For this review, take the finished solid that the model builds, in its own axes (mm). A direction names the side the tool comes from. Give positions to 0.01 mm unless a question says otherwise; leave off trailing zeros. Order: outer loops, then holes, each group sorted by start corner. A loop starts at its lowest first (then second) coordinate and runs counter-clockwise, first axis right, second up. Notation, with made-up numbers: (-17.5, 39.5) - (15.5, 39.5) arc R15 ccw to (15.5, 59.5) - close; hole circle Ø8 at (89, 20). An arc over 180 degrees is marked (long way). One line per item, written item: value.
```python
from build123d import *

# Parameters (mm, degrees)
BOSS_EXTRUDE1_DEPTH = 38.1
CUT_EXTRUDE1_DEPTH  = 98.457965419
SHELL1_START        = -38.1
SHELL1_DEPTH        = 75.35333418
FILLET1_R           = 17.78


# Read off the part's stored shape, not the designer's step: Shell1
with BuildPart() as part:
    # Sketch1 → Boss-Extrude1 (new, symmetric)
    with BuildSketch(Plane.XY):
        Polygon((-33.198119966, 25.4), (-33.198119966, -25.4), (33.198119966, -50.887128572), (33.198119966, -0.087128572), align=None)
    extrude(amount=BOSS_EXTRUDE1_DEPTH, both=True)

    # Sketch2 → Cut-Extrude1 (cut, through all)
    with BuildSketch(Plane.XY.offset(38.1)):
        Polygon((16.599059983, -44.515346429), (33.198119966, -33.107128572), (33.198119966, -50.887128572), align=None)
        Polygon((-16.599059983, 19.028217857), (-33.198119966, 25.4), (-33.198119966, 7.62), align=None)
    extrude(amount=-CUT_EXTRUDE1_DEPTH, mode=Mode.SUBTRACT)

    # Shell1 outline → Shell1 (cut)
    with BuildSketch(Plane.XY.offset(SHELL1_START)):
        Polygon((31.928119966, -0.506523102), (-16.486612201, 18.078151343), (-32.351454146, 7.174547563), (-32.351454146, -24.818102704), (16.486612201, -43.565279915), (31.928119966, -32.952625656), align=None)
    extrude(amount=SHELL1_DEPTH, mode=Mode.SUBTRACT)

    # Fillet1
    # the kernel refuses this fillet: 17.78 mm, written as the material it adds along each edge
    with BuildSketch(Plane(origin=(-14.571454146, -2.179962965, 19.47333418), x_dir=(-0.5664062369240325, 0.8241261886225658, 0), z_dir=(0, 0, 1))) as fillet1_piece_1_section:
        Polygon((0, 0), (FILLET1_R * 1.02, 0), (FILLET1_R * 1.02, FILLET1_R * 0.536647960523), (FILLET1_R * 0.577734361663, FILLET1_R * 0.840608712395), align=None)
    fillet1_piece_1 = extrude(amount=FILLET1_R * 1.02, mode=Mode.PRIVATE)
    fillet1_piece_1 = fillet1_piece_1 - Plane(origin=(-14.571454146, -2.179962965, 19.47333418), x_dir=(0.8849876374628157, -0.4656145203255411, 0), z_dir=(0, 0, 1)) * Sphere(FILLET1_R, mode=Mode.PRIVATE)
    add(fillet1_piece_1)
    with BuildSketch(Plane(origin=(-14.571454146, -12.59824726, 19.47333418), x_dir=(-1, 0, 0), z_dir=(0, 0, 1))) as fillet1_piece_2_section:
        Polygon((0, 0), (FILLET1_R * 1.02, 0), (FILLET1_R * 1.02, FILLET1_R * 0.701026577777), (FILLET1_R * 0.365535308531, FILLET1_R * 0.952252035029), align=None)
    fillet1_piece_2 = extrude(amount=FILLET1_R * 1.02, mode=Mode.PRIVATE)
    fillet1_piece_2 = fillet1_piece_2 - Plane(origin=(-14.571454146, -12.59824726, 19.47333418), x_dir=(0.8241261886205663, 0.5664062369269417, 0), z_dir=(0, 0, 1)) * Sphere(FILLET1_R, mode=Mode.PRIVATE)
    add(fillet1_piece_2)
    with BuildSketch(Plane(origin=(14.148119966, -12.726378546, 19.47333418), x_dir=(0.35836794954893786, 0.9335804264958054, 0), z_dir=(0, 0, 1))) as fillet1_piece_3_section:
        Polygon((0, 0), (FILLET1_R * 1.02, 0), (FILLET1_R * 1.02, -FILLET1_R * 0.701026577771), (FILLET1_R * 0.36553530854, -FILLET1_R * 0.952252035026), align=None)
    fillet1_piece_3 = extrude(amount=FILLET1_R * 1.02, mode=Mode.PRIVATE)
    fillet1_piece_3 = fillet1_piece_3 - Plane(origin=(14.148119966, -12.726378546, 19.47333418), x_dir=(-0.824126188623119, -0.5664062369232272, 0), z_dir=(0, 0, 1)) * Sphere(FILLET1_R, mode=Mode.PRIVATE)
    add(fillet1_piece_3)
    with BuildSketch(Plane(origin=(-14.125206416, -1.873265397, 19.47333418), x_dir=(0.35836794954893786, 0.9335804264958054, 0), z_dir=(0, 0, 1))) as fillet1_piece_4_section:
        Polygon((0, 0), (FILLET1_R * 1.02, 0), (FILLET1_R * 1.02, FILLET1_R * 0.536647960524), (FILLET1_R * 0.577734361661, FILLET1_R * 0.840608712396), align=None)
    fillet1_piece_4 = extrude(amount=FILLET1_R * 1.02, mode=Mode.PRIVATE)
    fillet1_piece_4 = fillet1_piece_4 - Plane(origin=(-14.125206416, -1.873265397, 19.47333418), x_dir=(0.11753739745542074, -0.9930684569552123, 0), z_dir=(0, 0, 1)) * Sphere(FILLET1_R, mode=Mode.PRIVATE)
    add(fillet1_piece_4)
    with BuildSketch(Plane(origin=(-32.351454146, -2.179962965, 37.25333418), x_dir=(0, 0, -1), z_dir=(0, -1, 0))) as fillet1_piece_5:
        with BuildLine():
            CenterArc((FILLET1_R, FILLET1_R), FILLET1_R, 180, 90)
            Line((0, FILLET1_R), (0, 0))
            Line((0, 0), (FILLET1_R, 0))
        make_face()
    extrude(amount=10.418284295)
    with BuildSketch(Plane(origin=(-20.943236289, -29.197307243, 37.25333418), x_dir=(0, 0, -1), z_dir=(0.9335804264990358, -0.3583679495405224, 0))) as fillet1_piece_6_section:
        with BuildLine():
            CenterArc((FILLET1_R, FILLET1_R), FILLET1_R, 180, 90)
            Line((0, FILLET1_R), (0, 0))
            Line((0, 0), (FILLET1_R, 0))
        make_face()
    fillet1_piece_6 = extrude(amount=84.542794822, mode=Mode.PRIVATE)
    fillet1_piece_6 = split(fillet1_piece_6, bisect_by=Plane(origin=(10.612775851, -47.602255792, 33.386694553), z_dir=(-0.5664062369254325, 0.8241261886216036, 0)), keep=Keep.TOP, mode=Mode.PRIVATE)
    fillet1_piece_6 = split(fillet1_piece_6, bisect_by=Plane(origin=(31.928119966, -33.018136408, 33.386694553), z_dir=(-1, 0, 0)), keep=Keep.TOP, mode=Mode.PRIVATE)
    add(fillet1_piece_6)
    with BuildSketch(Plane(origin=(31.928119966, -77.402625656, 37.25333418), x_dir=(0, 0, -1), z_dir=(0, 1, 0))) as fillet1_piece_7_section:
        with BuildLine():
            CenterArc((FILLET1_R, FILLET1_R), FILLET1_R, 180, 90)
            Line((0, FILLET1_R), (0, 0))
            Line((0, 0), (FILLET1_R, 0))
        make_face()
    fillet1_piece_7 = extrude(amount=64.67624711, mode=Mode.PRIVATE)
    fillet1_piece_7 = split(fillet1_piece_7, bisect_by=Plane(origin=(19.754469789, -44.819692915, 33.477432333), z_dir=(0.3583679495405224, 0.9335804264990358, 0)), keep=Keep.TOP, mode=Mode.PRIVATE)
    fillet1_piece_7 = split(fillet1_piece_7, bisect_by=Plane(origin=(33.035848264, -32.191305089, 33.477432333), z_dir=(-0.5664062369254325, 0.8241261886216036, 0)), keep=Keep.TOP, mode=Mode.PRIVATE)
    add(fillet1_piece_7)
    with BuildSketch(Plane(origin=(-32.351454146, -24.818102704, -38.1), x_dir=(0, 1, 0), z_dir=(0, 0, 1))) as fillet1_piece_8:
        with BuildLine():
            CenterArc((FILLET1_R * 0.687280958605, -FILLET1_R), FILLET1_R, 90, 69)
            Line((-FILLET1_R * 0.246299467894, -FILLET1_R * 0.641632050459), (0, 0))
            Line((0, 0), (FILLET1_R * 0.687280958605, 0))
        make_face()
    extrude(amount=57.57333418)
    with BuildSketch(Plane(origin=(-32.351454146, 7.174547563, -38.1), x_dir=(0.8241261886225659, 0.5664062369240322, 0), z_dir=(0, 0, 1))) as fillet1_piece_9:
        with BuildLine():
            CenterArc((FILLET1_R * 0.526125451493, -FILLET1_R), FILLET1_R, 90, 55.5)
            Line((-FILLET1_R * 0.29800073713, -FILLET1_R * 0.433593763076), (0, 0))
            Line((0, 0), (FILLET1_R * 0.526125451493, 0))
        make_face()
    extrude(amount=57.57333418)
    with BuildSketch(Plane(origin=(16.486612201, -43.565279915, -38.1), x_dir=(-0.933580426499036, 0.3583679495405219, 0), z_dir=(0, 0, 1))) as fillet1_piece_10:
        with BuildLine():
            CenterArc((FILLET1_R * 0.526125451489, -FILLET1_R), FILLET1_R, 90, 55.5)
            Line((-FILLET1_R * 0.29800073713, -FILLET1_R * 0.433593763072), (0, 0))
            Line((0, 0), (FILLET1_R * 0.526125451489, 0))
        make_face()
    extrude(amount=75.35333418)
    with BuildSketch(Plane(origin=(31.928119966, -32.952625656, -38.1), x_dir=(-0.8241261886216035, -0.5664062369254323, 0), z_dir=(0, 0, 1))) as fillet1_piece_11:
        with BuildLine():
            CenterArc((FILLET1_R * 0.526125451492, -FILLET1_R), FILLET1_R, 90, 55.5)
            Line((-FILLET1_R * 0.29800073713, -FILLET1_R * 0.433593763075), (0, 0))
            Line((0, 0), (FILLET1_R * 0.526125451492, 0))
        make_face()
    extrude(amount=75.35333418)
    with BuildSketch(Plane(origin=(-16.486612201, 18.078151343, -38.1), x_dir=(0.9335804264958054, -0.35836794954893825, 0), z_dir=(0, 0, 1))) as fillet1_piece_12:
        with BuildLine():
            CenterArc((FILLET1_R * 0.526125451494, -FILLET1_R), FILLET1_R, 90, 55.5)
            Line((-FILLET1_R * 0.29800073713, -FILLET1_R * 0.433593763078), (0, 0))
            Line((0, 0), (FILLET1_R * 0.526125451494, 0))
        make_face()
    extrude(amount=57.57333418)
    with BuildSketch(Plane(origin=(31.928119966, -0.506523102, -38.1), x_dir=(-0.9335804264958055, 0.3583679495489376, 0), z_dir=(0, 0, 1))) as fillet1_piece_13:
        with BuildLine():
            CenterArc((FILLET1_R * 0.687280958599, FILLET1_R), FILLET1_R, 201, 69)
            Line((-FILLET1_R * 0.246299467897, FILLET1_R * 0.641632050451), (0, 0))
            Line((0, 0), (FILLET1_R * 0.687280958599, 0))
        make_face()
    extrude(amount=57.57333418)
    with BuildSketch(Plane(origin=(20.519902109, 3.872681437, 37.25333418), x_dir=(0, 0, -1), z_dir=(-0.9335804264958054, 0.35836794954893786, 0))) as fillet1_piece_14:
        with BuildLine():
            CenterArc((FILLET1_R, FILLET1_R), FILLET1_R, 180, 90)
            Line((0, FILLET1_R), (0, 0))
            Line((0, 0), (FILLET1_R, 0))
        make_face()
    extrude(amount=30.284832008)
    with BuildSketch(Plane(origin=(-24.195909309, 12.779698237, 37.25333418), x_dir=(0, 0, -1), z_dir=(-0.8241261886225658, -0.5664062369240325, 0))) as fillet1_piece_15:
        with BuildLine():
            CenterArc((FILLET1_R, FILLET1_R), FILLET1_R, 180, 90)
            Line((0, FILLET1_R), (0, 0))
            Line((0, 0), (FILLET1_R, 0))
        make_face()
    extrude(amount=0.541479856)


solid = part.part
```
(1) For P1, Ø10, axis at x = -16.5, y = -3, coming from the -Z side; P2, Ø17.5, axis at x = -4, y = -10, coming from the -Z side; P3, Ø2, axis at x = -20.5, z = 18.5, coming from the -Y side; P4, Ø10, axis at x = 14, y = 5, coming from the -Z side, all flat-tipped, find the tip position at first contact; note any pin that passes through.
Answers below:
P1: stops at z = 35.85
P2: stops at z = 36.6
P3: stops at y = -30.66
P4: stops at z = -38.1
(2) Draft analysis for pull direction X (two halves, no side actions). For faces 1 (the face through (31.928, -18, -10)), 2 (the face through (24.782, -38.891, 0.533)), 3 (the face through (0, -12, 38.1)), state which applies: pulls with the +X half, pulls with the -X half, needs draft (parallel to the pull), parting line crosses it, or undercut.
Answers below:
face 1: undercut
face 2: pulls with the +X half
face 3: needs draft
(3) Wall thickness on line 1 (Y direction, x = 0, z = 33); line 2 (X direction, y = -11.5, z = 4.5); line 3 (Y direction, x = -2, z = -23.5): over which ranges is each line inside the solid? List them lowest first. Write a range as from..to.
Answers below:
line 1: y = -38.14..-30.55, 5.06..12.66
line 2: x = -33.2..-32.35, 31.89..33.2
line 3: y = -37.38..-36.47, 12.52..13.42
(4) Machinability: for faces 4 (the face through (-32.351, -7, -10)), 5 (the face through (-8.648, -34.824, 0.533)), which of the approach directions +Z, -Z, +X, -X, +Y, -Y give a long, thin tool a straight path to every point of the face, cutting with its end or side? Answer none if there is none.
Answers below:
face 4: -Z
face 5: +Z, -Z, -X, -Y
(5) Take a section at B-B (x = 26). Write out the cut boundary in (y, z), then the cut area to 3 significant figures.
Answers below:
outline: (-38.05, -38.1) - (-36.85, -38.1) - (-36.85, 32.73) - (-12.73, 32.73) arc R13.25 cw to (0.53, 19.47) - (0.53, -38.1) - (2.68, -38.1) - (2.68, 38.1) - (-38.05, 38.1) - close
area: 494 mm^2
